Geometry: final body of the model. Coordinates: model frame, mm. A direction names the side the tool comes from. Round coordinates to 2 decimals unless told otherwise and drop trailing zeros. Order: outer loops, then holes, each group sorted by start corner. A loop starts at its lowest first (then second) coordinate and runs counter-clockwise, first axis right, second up. Notation, with made-up numbers: M -24.75,-34.5 L 16.25,-34.5 A23 cw 16.25,-22.5 Z; hole C 67,37.5 d3. An arc over 180 degrees is marked long. Return JSON: item names as keys, results as strings. Group by question number.
Q1. Access query for faces 1 (the face through (3, 125.7, 6)), 2 (the face through (-3.76, 62, 0)). Directions: +Z, -Z, +X, -X, +Y, -Y. A direction counts if a zero-diameter tool reaches every point of the face in a straight line with its end or side. Return the directions, or none.
Q2. Cut plane A-A on y = 43. Output: boundary loops of the cut face in (x, z), and give its area (3 significant figures).
Q3. Mould query, pull axis X, two halves, no side actions, for faces 3 (the face through (1, 62, 5)), 4 (the face through (-7.364, 61.97, -3.062)), 5 (the face through (0, 62, 7)). Classes: released by +X, released by -X, zero draft, split by the parting line, or undercut.
Q4. Cut plane B-B on z = 1.75. Output: boundary loops of the cut face in (x, y), and give its area (3 significant figures).
Q5. Cut plane D-D on x = -7. Output: boundary loops of the cut face in (y, z), and give its area (3 significant figures).
Q6. Contact query for flat-ended pins moving along their axis: pin 1 (12 mm diameter, centred on x = -7, y = 66.5, fed in from -Z); pin 2 (5 mm diameter, centred on x = 0, y = 77, fed in from -Z); pin 3 (12 mm diameter, centred on x = -8.5, y = 76.5, fed in from -Z) (3 decimals). Output: stop coordinate, or through.
Q7. Ray query, probe 1 along Z at (x, y) = (3.5, 27); probe 2 along X at (y, z) = (98, -3); probe 3 along X at (y, z) = (59, -4.75). Return the intervals inside material, ascending.
Q8. Cut plane C-C on x = 1. Output: boundary loops of the cut face in (y, z), and give its area (3 significant figures).
```python
from build123d import *

# Parameters (mm, degrees)
SKETCH_1_W          = 24.4
SKETCH_1_H          = 14
EXTRUDE_1_DEPTH     = 125.7
CUT_EXTRUDE_1_DEPTH = 125.7
FILLET_1_R          = 15


with BuildPart() as part:
    # Эскиз1 → Бобышка-Вытянуть1 (new body)
    with BuildSketch(Plane(origin=(0, 0, 0), x_dir=(1, 0, 0), z_dir=(0, 1, 0))):
        Rectangle(SKETCH_1_W, SKETCH_1_H)
    extrude(amount=EXTRUDE_1_DEPTH)

    # Эскиз5 → Вырез-Вытянуть1 (cut)
    with BuildSketch(Plane(origin=(0, 0, 0), x_dir=(-1, 0, 0), z_dir=(0, -1, 0))):
        Polygon((-1.24, 0), (-1.24, -5), (3.76, -5), (3.76, 5), (-1.234412321, 5), (0, 0), align=None)
        Polygon((-6.24, -5), (-1.24, -5), (-1.24, 0), (-1.24, 5), (-6.24, 5), align=None)
        Polygon((-1.24, 5), (-1.24, 0), (0, 0), (-1.234412321, 5), align=None)
    extrude(amount=-CUT_EXTRUDE_1_DEPTH, mode=Mode.SUBTRACT)

    # Скругление1
    # the kernel refuses this fillet: 15 mm, written as the material it takes off along each edge
    with BuildSketch(Plane(origin=(-12.2, -37.416573868, -7), x_dir=(1, 0, 0), z_dir=(0, 1, 0))) as fillet_1_piece_1:
        with BuildLine():
            CenterArc((14.966629547, -15), FILLET_1_R, 90, 86.177446271)
            Line((0, -14), (-0.299332591, -13.98))
            ThreePointArc((-0.299332591, -13.98), (-0.3, -7), (-0.3, 0))
            Line((-0.3, 0), (0, 0.3))
            Line((0, 0.3), (14.966629547, 0.3))
            Line((14.966629547, 0.3), (14.966629547, 0))
        make_face()
    extrude(amount=200.533147735, mode=Mode.SUBTRACT)


solid = part.part
```
Result sheet:
{
 "1": {"face 1": "+Z, -Z, +X, -X, +Y", "face 2": "+Y, -Y"},
 "2": {"outline": "M -12.2,7 A15 ccw 2.77,-7 L 12.2,-7 L 12.2,7 Z; hole M -3.76,-5 L 6.24,-5 L 6.24,5 L -3.76,5 Z", "area": "194 mm²"},
 "3": {"face 3": "undercut", "face 4": "released by -X", "face 5": "zero draft"},
 "4": {"outline": "M -10.87,0 L -3.76,0 L -3.76,125.7 L -10.87,125.7 Z; M 6.24,0 L 12.2,0 L 12.2,125.7 L 6.24,125.7 Z", "area": "1,640 mm²"},
 "5": {"outline": "M 0,-3.38 L 125.7,-3.38 L 125.7,7 L 0,7 Z", "area": "1,310 mm²"},
 "6": {"pin 1": "stops at z = -6.52", "pin 2": "stops at z = -7", "pin 3": "stops at z = -6.045"},
 "7": {"probe 1": "z = -7 to -5, 5 to 7", "probe 2": "x = -7.43 to -3.76, 6.24 to 12.2", "probe 3": "x = -5.14 to -3.76, 6.24 to 12.2"},
 "8": {"outline": "M 0,-6.9 L 125.7,-6.9 L 125.7,-5 L 0,-5 Z; M 0,5 L 125.7,5 L 125.7,7 L 0,7 Z", "area": "490 mm²"}
}
